The model under review builds one solid part; all positions refer to its coordinate system, in mm. A direction names the side the tool comes from. Give positions to 0.01 mm unless a question says otherwise; leave off trailing zeros. Loops run counter-clockwise (first coordinate to the right, second up) from the corner with the lowest first, then second, coordinate; pieces in that order, holes last. Notation, with made-up numbers: (-10.5, -9.75) - (6.5, -9.75) arc R31 ccw to (6.5, 25.25) - close; hole circle Ø5 at (38, -19). An arc over 180 degrees is marked (long way). Return JSON: item names as keys, results as strings. Group by question number.
```python
from build123d import *

# Parameters (mm, degrees)
F1_DEPTH = 152.4
F2_W     = 101.6
F2_H     = 76.2
F3_DEPTH = 76.2
F5_DEPTH = 76.2
F7_D     = 9.525
F9_D     = 12.7


with BuildPart() as f1:
    # F0 (on Front) → F1 (new body)
    with BuildSketch(Plane.XZ):
        Polygon((13.440086, 20.999823), (13.440086, 173.399823), (-37.359914, 173.399823), (-37.359914, -29.800177), (115.040086, -29.800177), (115.040086, 20.999823), align=None)
    extrude(amount=F1_DEPTH)

    # F2 (on face) → F3 (join)
    with BuildSketch(Plane.XY.offset(20.999823)):
        with Locations((50.8, -38.1)):
            Rectangle(F2_W, F2_H)
    extrude(amount=F3_DEPTH)

    # F4 (on face) → F5 (cut)
    with BuildSketch(Plane.XZ.offset(76.2)):
        Polygon((101.6, 97.199823), (13.440086, 97.199823), (101.6, 20.999823), align=None)
    extrude(amount=-F5_DEPTH, mode=Mode.SUBTRACT)

    # F7 (through all)
    with Locations(Plane.XY.offset(20.999823)):
        with Locations((76.940086, -114.3)):
            Hole(F7_D / 2)

    # F9 (through all)
    with Locations(Plane.YZ.offset(13.440086)):
        with Locations((-114.3, 135.299823)):
            Hole(F9_D / 2)


solid = f1.part
```
1) For pin 1 Ø6 at (x, y) = (85, -51.5) entering from +Z; pin 2 Ø4 at (y, z) = (-89.5, 144) entering from +X; pin 3 Ø15 at (x, y) = (76.94, -114.3) entering from +Z, all flat-tipped, find the tip position at first contact; note any pin that passes through.
2) Draft analysis for pull direction Y (two halves, no side actions). For faces 1 (the face through (4, -152.4, 51)), 2 (the face through (77.97, -118.95, -4.76)), 3 (the face through (38, -75, -29.8)), state which applies: +Y half, -Y half, draft (parallel to the pull), parting line (faces both ways), or undercut.
3) To check wall thickness, follow line 1 (Z direction, x = -10, y = -114.3); line 2 (X direction, y = -114, z = 8); line 3 (Z direction, x = 99.5, y = -142). State the ranges of each line that lie inside material, in increasing order.
4) Tool access review of faces 4 (the face through (65, -109, 21)), 5 (the face through (21, 0, 51)): name each direction out of +Z, -Z, +X, -X, +Y, -Y from which nothing blocks a thin tool from reaching the whole face with its end or side.
5) We need section A-A, the plane y = -114.3. Write out the cut boundary in (x, z).
6) We need section C-C, the plane z = 76. Write out the cut boundary in (x, y).
7) We need section D-D, the plane y = -16. Write out the cut boundary in (x, z), plus the area to 3 significant figures.
8) We need section B-B, the plane y = -87. Write out the cut boundary in (x, z).
Findings:
{
 "1": {"pin 1": "stops at z = 37.94", "pin 2": "stops at x = 13.44", "pin 3": "stops at z = 21"},
 "2": {"face 1": "-Y half", "face 2": "undercut", "face 3": "draft"},
 "3": {"line 1": "z = -29.8 to 128.95, 141.65 to 173.4", "line 2": "x = -37.36 to 72.19, 81.69 to 115.04", "line 3": "z = -29.8 to 21"},
 "4": {"face 4": "+Z, +X, -Y", "face 5": "+Z, -Z, +X, -X, +Y"},
 "5": {"outline": "(-37.36, -29.8) - (72.18, -29.8) - (72.18, 21) - (13.44, 21) - (13.44, 128.95) - (-37.36, 128.95) - close; (-37.36, 141.65) - (13.44, 141.65) - (13.44, 173.4) - (-37.36, 173.4) - close; (81.7, -29.8) - (115.04, -29.8) - (115.04, 21) - (81.7, 21) - close"},
 "6": {"outline": "(-37.36, -152.4) - (13.44, -152.4) - (13.44, -76.2) - (37.97, -76.2) - (37.97, 0) - (-37.36, 0) - close"},
 "7": {"outline": "(-37.36, -29.8) - (115.04, -29.8) - (115.04, 21) - (101.6, 21) - (13.44, 97.2) - (13.44, 173.4) - (-37.36, 173.4) - close", "area": "18,800 mm^2"},
 "8": {"outline": "(-37.36, -29.8) - (115.04, -29.8) - (115.04, 21) - (13.44, 21) - (13.44, 173.4) - (-37.36, 173.4) - close"}
}
